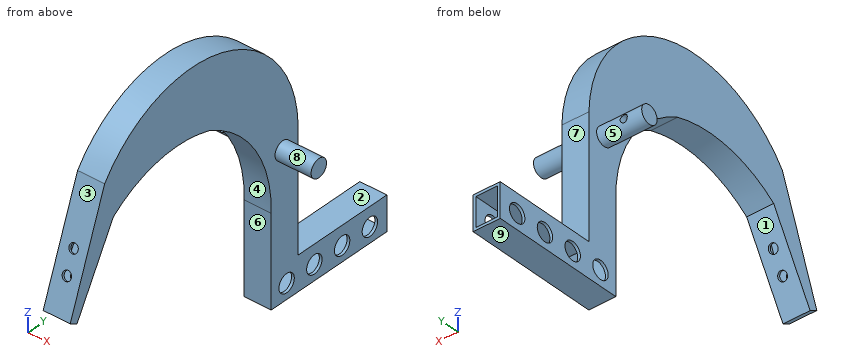
```python
from build123d import *

# Parameters (mm, degrees)
BOSS_EXTRUDE1_DEPTH = 15
SHELL1_START        = -12
SHELL1_DEPTH        = 24
SKETCH3_R           = 10
CUT_EXTRUDE2_DEPTH  = 412.603799071
BOSS_EXTRUDE2_START = 40
SKETCH4_R           = 10
BOSS_EXTRUDE2_DEPTH = 120
LPATTERN1_COUNT     = 4
LPATTERN1_PITCH     = 36
SKETCH6_R           = 5
CUT_EXTRUDE3_DEPTH  = 416.623251767
CUT_EXTRUDE4_REACH  = 417.623
SKETCH7_R           = 4


# Read off the part's stored shape, not the designer's step: Shell1
with BuildPart() as part:
    # Sketch1 → Boss-Extrude1 (new, symmetric)
    with BuildSketch(Plane(origin=(0, 0, 0), x_dir=(0, 0, -1), z_dir=(1, 0, 0))):
        with BuildLine():
            Line((0, 0), (85.251371582, -47.255606917))
            Line((85.251371582, -47.255606917), (80.40327538, -56.001803988))
            Line((80.40327538, -56.001803988), (-40.245063676, -11.361449965))
            ThreePointArc((-40.245063676, -11.361449965), (-93.575565654, 141.17838747), (34.587469981, 239.599831994))
            Line((34.587469981, 239.599831994), (168.825159395, 239.599831994))
            Line((168.825159395, 239.599831994), (168.825159395, 354.599831994))
            Line((168.825159395, 354.599831994), (206.825159395, 354.599831994))
            Line((206.825159395, 354.599831994), (206.825159395, 204.599831994))
            Line((206.825159395, 204.599831994), (106.825159395, 204.599831994))
            ThreePointArc((106.825159395, 204.599831994), (30.408436566, 184.017865838), (-21.845490063, 124.581611838))
            ThreePointArc((-21.845490063, 124.581611838), (-26.384125187, 59.579639949), (0, 0))
        make_face()
    extrude(amount=BOSS_EXTRUDE1_DEPTH, both=True)

    # Shell1 outline → Shell1 (cut)
    with BuildSketch(Plane.YZ.offset(SHELL1_START)):
        with BuildLine():
            ThreePointArc((125.505371341, 24.69972698), (125.667778254, 24.641959892), (125.826599381, 24.574960703))
            ThreePointArc((125.826599381, 24.574960703), (186.553407601, -28.804836135), (207.599831994, -106.870164943))
            Line((207.599831994, -106.870164943), (207.599831994, -203.825159395))
            Line((207.599831994, -203.825159395), (354.599831994, -203.825159395))
            Line((354.599831994, -203.825159395), (354.599831994, -171.825159395))
            Line((354.599831994, -171.825159395), (236.599831994, -171.825159395))
            Line((236.599831994, -171.825159395), (236.599831994, -34.630851514))
            ThreePointArc((236.599831994, -34.630851514), (140.483066901, 90.652257864), (-8.681515002, 38.842823077))
            Line((-8.681515002, 38.842823077), (-52.294295287, -79.028318808))
            Line((-52.294295287, -79.028318808), (-48.425037178, -81.1730836))
            Line((-48.425037178, -81.1730836), (-2.327347545, 1.989349905))
            ThreePointArc((-2.327347545, 1.989349905), (58.757023973, 29.285300463), (125.505371341, 24.69972698))
        make_face()
    extrude(amount=SHELL1_DEPTH, mode=Mode.SUBTRACT)

    # Sketch3 → Cut-Extrude2 (cut, through all)
    with BuildSketch(Plane(origin=(15, 0, 0), x_dir=(0, 0, -1), z_dir=(1, 0, 0))):
        with Locations((189.825159395, 224.599831994)):
            Circle(SKETCH3_R)
    cut_extrude2 = extrude(amount=-CUT_EXTRUDE2_DEPTH, mode=Mode.SUBTRACT)

    # Sketch4 → Boss-Extrude2 (add)
    with BuildSketch(Plane(origin=(15, 0, 0), x_dir=(0, 0, -1), z_dir=(1, 0, 0)).offset(BOSS_EXTRUDE2_START)):
        with Locations((49.825159395, 219.599831994)):
            Circle(SKETCH4_R)
    extrude(amount=-BOSS_EXTRUDE2_DEPTH)

    # LPattern1: Cut-Extrude2 ×4
    with Locations(*[(0, i * LPATTERN1_PITCH, 0) for i in range(1, LPATTERN1_COUNT)]):
        add(cut_extrude2, mode=Mode.SUBTRACT)

    # Sketch6 → Cut-Extrude3 (cut, through all)
    with BuildSketch(Plane(origin=(0, 0, 0), x_dir=(1, 0, 0), z_dir=(0, 0.8746197071393954, -0.48480962024633795))):
        with Locations(Location((0, 35, 0), (0, 0, 270))):
            Circle(SKETCH6_R)
        with Locations(Location((0, 60, 0), (0, 0, 270))):
            Circle(SKETCH6_R)
    extrude(amount=-CUT_EXTRUDE3_DEPTH, mode=Mode.SUBTRACT)

    # Sketch7 → Cut-Extrude4 (cut, up to next)
    with BuildSketch(Plane(origin=(0, 0, 0), x_dir=(1, 0, 0), z_dir=(0, 1, 0)), mode=Mode.PRIVATE) as cut_extrude4_sk1:
        with Locations(Location((-45, 49.825159395, 0), (0, 0, 90))):
            Circle(SKETCH7_R)
    cut_extrude4_tool1 = extrude(cut_extrude4_sk1.sketch, amount=CUT_EXTRUDE4_REACH, mode=Mode.PRIVATE) & part.part
    add(cut_extrude4_tool1.solids().sort_by_distance((-45, 0, -49.825159))[0], mode=Mode.SUBTRACT)


solid = part.part
```
Can you work these out from the model? Positions are in its coordinate system, mm. Face numbers are marked on the shaded views. A direction names the side the tool comes from. Coordinates: 2 decimals unless noted, no trailing zeros. Write each loop counter-clockwise with the first axis right and the second up, starting at its lowest first coordinate (ties: lowest second). Pieces come first, ordered by that corner, then holes. Notation, with made-up numbers: (75.25, 20.25) - (83.25, 20.25) arc R24 cw to (83.25, 52.25) - close; hole circle Ø1 at (75.5, 65). An arc over 180 degrees is marked (long way). Return JSON: item names as keys, results as strings.
Q1. On a 3-axis mill with a long thin cutter (end or side, diameter ignored), from which of +Z, -Z, +X, -X, +Y, -Y can I reach the whole of each face in a straight line? I mean the marked faces 5, 6, 7, 8 and 9. Say none if no direction works.
Computed values:
{"face 5": "-X", "face 6": "-Z, +X, -X, -Y", "face 7": "+Z, +X, -X, +Y", "face 8": "+X", "face 9": "-Z, +X, -X, +Y, -Y"}
Q2. If we section it at D-D (z = 51.5): Please give me the cut outline in (x, y).
Computed values:
{"outline": "(-15, -2.63) - (15, -2.63) - (15, 206.19) - (-15, 206.19) - close; hole (-12, 1.37) - (12, 1.37) - (12, 202.19) - (-12, 202.19) - close"}
Q3. If we section it at C-C (x = -54.5): Please give me the cut outline in (y, z).
Computed values:
{"outline": "circle Ø20 at (219.6, -49.83)"}
Q4. I'm going to push flat-ended pins straight in: pin 1 Ø16 at (y, z) = (260.6, -189.83) entering from -X; pin 2 Ø4 at (x, y) = (3, 220) entering from +Z; pin 3 Ø24 at (x, z) = (-5.5, -126) entering from +Y; pin 4 Ø23 at (y, z) = (296.6, -189.83) entering from -X. Where does each tip first touch, or does it pass through?
Computed values:
{"pin 1": "passes through", "pin 2": "stops at z = 35.63", "pin 3": "stops at y = 239.6", "pin 4": "stops at x = -15"}
Q5. Thinking about a two-plate mould opening in Y: for the marked faces 1, 2, 3 and 4, which applies, +Y half, -Y half, draft (parallel to the pull), parting line (faces both ways), or undercut?
Computed values:
{"face 1": "undercut", "face 2": "draft", "face 3": "-Y half", "face 4": "undercut"}
Q6. Please list where these lines run through material, in increasing order: L1, parallel to Y at x = 4, z = -143; L2, parallel to X at y = 249, z = -173; L3, parallel to Z at x = 2.5, y = 85. Write a range as from..to.
Computed values:
{"L1": "y = 204.6..207.6, 236.6..239.6", "L2": "x = -15..-12, 12..15", "L3": "z = 28.4..31.4, 95.28..98.3"}
Q7. If we section it at A-A (z = 13): Please give me the cut outline in (x, y).
Computed values:
{"outline": "(-15, -21.44) - (15, -21.44) - (15, 20.23) - (-15, 20.23) - close; (-15, 140.93) - (15, 140.93) - (15, 229.66) - (-15, 229.66) - close; hole (-12, -18.24) - (12, -18.24) - (12, 14) - (-12, 14) - close; hole (-12, 146.4) - (12, 146.4) - (12, 226.42) - (-12, 226.42) - close"}
Q8. If we section it at B-B (z = -139): Please give me the cut outline in (x, y), then the cut area to 3 significant figures.
Computed values:
{"outline": "(-15, 204.6) - (15, 204.6) - (15, 239.6) - (-15, 239.6) - close; hole (-12, 207.6) - (12, 207.6) - (12, 236.6) - (-12, 236.6) - close", "area": "354 mm2"}
